Autodesk Fusion 360 part; units mm, degrees
sketch "Sketch1" plane through (0, 0, 0) normal (0, 0, 1) x (1, 0, 0)
  circle A0 centre (0, 0) radius 65
  dimension "d1" = 130
extrude "Extrude1" add sketch "Sketch1" along normal blind 60
hole "Hole1" at (0, 0, 60) direction (0, 0, -1) diameter 124 depth 55 tip angle 180
ref_plane "WorkPlane1" through (65, 0, 32.9588) normal (1, 0, 0) x (0, -1, 0)
ref_plane "WorkPlane2" through (77.5, 0, 32.9588) normal (1, 0, 0) x (0, -1, 0)
sketch "Sketch2" plane through (77.5, 0, 32.9588) normal (1, 0, 0) x (0, 1, 0)
  line L0 (-8, -8) -> (8, -8)
  line L1 (8, -8) -> (8, 18)
  line L2 (8, 18) -> (-8, 18)
  line L3 (-8, 18) -> (-8, -8)
  line L4 (-8, -8) -> (8, 18) construction
  line L5 (8, -8) -> (-8, 18) construction
  point P0 (0, 5)
  dimension "d9" = 16
extrude "Extrude2" add sketch "Sketch2" along normal up to surface end surface at (64.677, -6.4719, 40)
extrude "Extrude3" add 1 faces at (77.5, -2.6667, 33.6254) along direction (1, 0, 0) blind 0.5
extrude "Extrude4" cut 1 faces at (73.6667, 0, 24.9588) along direction (0, 0, 1) blind 1
extrude "Extrude5" add 1 faces at (78, -2.6667, 42.6254) along direction (1, 0, 0) blind 0.2
shell "Shell1" thickness 1 removed faces 2 at (69.0705, 8, 34.2921) at (73.8, 0, 50.9588)
ref_plane "WorkPlane3" through (49.7929, 41.7812, 24.979) normal (0.766, 0.6428, 0) x (0.6428, -0.766, 0)
sketch "Sketch3" plane through (49.7929, 41.7812, 24.979) normal (0.766, 0.6428, 0) x (0.6428, -0.766, 0)
  line L0 (20, -20) -> (-20, -20)
  line L1 (-20, -20) -> (-20, 10)
  line L2 (-20, 10) -> (20, 10)
  line L3 (20, 10) -> (20, -20)
  line L4 (20, -20) -> (-20, 10) construction
  line L5 (-20, -20) -> (20, 10) construction
  point P0 (0, -5)
  dimension "d20" = 40
extrude "Extrude6" cut sketch "Sketch3" against normal blind 20
fillet "Fillet1" radius 0.4 8 edges at (78.2, 0, 50.9588) (77.7, 8, 50.9588) (78.2, 8, 38.4588) (71.3529, 8, 25.9588) (78.2, 0, 25.9588) (78.2, -8, 38.4588) (71.3529, -8, 50.9588) (71.3529, -8, 25.9588)
fillet "Fillet2" radius 2 1 edges at (-60.6013, -23.505, 0)
ref_plane "WorkPlane4" through (49.7929, 41.7812, 24.979) normal (0.766, 0.6428, 0) x (0.6428, -0.766, 0)
ref_plane "WorkPlane5" through (-45.9619, -45.9619, 2.3267) normal (-0.7071, -0.7071, 0) x (-0.7071, 0.7071, 0)
ref_plane "WorkPlane6" through (-55.2958, -55.2958, 2.3267) normal (-0.7071, -0.7071, 0) x (-0.7071, 0.7071, 0)
sketch "Sketch4" plane through (-55.2958, -55.2958, 2.3267) normal (-0.7071, -0.7071, 0) x (-0.7071, 0.7071, 0)
  line L0 (13, -31.7116) -> (-13, -31.7116)
  line L1 (-13, -31.7116) -> (-13, -47.7116)
  line L2 (-13, -47.7116) -> (13, -47.7116)
  line L3 (13, -47.7116) -> (13, -31.7116)
  line L4 (13, -31.7116) -> (-13, -47.7116) construction
  line L5 (-13, -31.7116) -> (13, -47.7116) construction
  point P0 (0, -39.7116)
  dimension "d31" = 26
  dimension "d32" = 16
extrude "Extrude7" add sketch "Sketch4" along normal up to surface end surface at (62.1344, 19.0871, 28.7723)
extrude "Extrude8" cut 1 faces at (-52.2316, -58.3599, 39.3716) along direction (0.707107, 0.707107, 0) blind 0.5
shell "Shell2" thickness 1 removed faces 1 at (-52.9418, -50.8867, 50.0383)
Design review of the part built by this model. Coordinates are the model's own, in mm. A direction names the side the tool comes from. Round coordinates to 2 decimals unless told otherwise and drop trailing zeros. Write each loop counter-clockwise with the first axis right and the second up, starting at its lowest first coordinate (ties: lowest second). Pieces come first, ordered by that corner, then holes. Notation, with made-up numbers: (45.5, -7.75) -> (66.5, -7.75) arc R25 cw to (66.5, 11.25) -> close; hole circle Ø3 at (3, -13). An arc over 180 degrees is marked (long way). Answer in a Markdown table with one row per item.
Q1. Take a section at A-A, the plane y = 0. State the section outline as (x, z) points.
The answers:
| item | result |
|---|---|
| outline | (-65, 2) arc R2 ccw to (-63, 0) -> (63, 0) arc R2 ccw to (65, 2) -> (65, 25.96) -> (77.8, 25.96) arc R0.4 ccw to (78.2, 26.36) -> (78.2, 50.56) arc R0.4 ccw to (77.8, 50.96) -> (65, 50.96) -> (65, 60) -> (62, 60) -> (62, 5) -> (-62, 5) -> (-62, 60) -> (-65, 60) -> close |
Q2. Take a section at C-C, the plane x = 0. State the section outline as (y, z) points.
The answers:
| item | result |
|---|---|
| outline | (-65, 2) arc R2 ccw to (-63, 0) -> (63, 0) arc R2 ccw to (65, 2) -> (65, 60) -> (62, 60) -> (62, 5) -> (-62, 5) -> (-62, 60) -> (-65, 60) -> close |
Q3. Draft analysis for pull direction Y (two halves, no side actions). For faces 1 (the face through (71, 8, 38)), 2 (the face through (-1, 1, 5)), 3 (the face through (-59.25, -40.865, 42.15)), 4 (the face through (71, 0, 25.959)), state which applies: +Y half, -Y half, draft (parallel to the pull), parting line (faces both ways), or undercut.
The answers:
| item | result |
|---|---|
| face 1 | +Y half |
| face 2 | undercut |
| face 3 | undercut |
| face 4 | draft |
Q4. Clearance check with flat-ended pins moving along their axes: pin 1 Ø10 at (y, z) = (20, 19) entering from +X; pin 2 Ø4 at (x, z) = (72, 43) entering from -Y; pin 3 Ø3 at (y, z) = (-18.5, 42) entering from -X. State where each tip first meets the part, or that it passes through.
The answers:
| item | result |
|---|---|
| pin 1 | x = 63.25 |
| pin 2 | y = -8 |
| pin 3 | x = -62.74 |
Q5. For faces 5 (the face through (-40.865, -59.25, 41.926)), 6 (the face through (-50, -50, 50.038)), 7 (the face through (71, -8, 39)), list the 3-axis set-ups (+Z, -Z, +X, -X, +Y, -Y) from which the entire face can be reached by the end or side of a thin tool; tool diameter is ignored.
The answers:
| item | result |
|---|---|
| face 5 | +Z, -Z, -Y |
| face 6 | +Z, -X, -Y |
| face 7 | +Z, -Z, +X, -Y |
Q6. To check wall thickness, follow L1, parallel to Y at x = 0, z = 30; L2, parallel to Z at x = -15, y = 0. State the ranges of each line that lie inside material, in increasing order. Write a range as [from, to].
The answers:
| item | result |
|---|---|
| L1 | [-65, -62], [62, 65] |
| L2 | [0, 5] |
Q7. Take a section at D-D, the plane z = 56. State the section outline as (x, y) points.
The answers:
| item | result |
|---|---|
| outline | circle Ø130 at (0, 0); hole circle Ø124 at (0, 0) |
Q8. Take a section at B-B, the plane z = 40. State the section outline as (x, y) points.
The answers:
| item | result |
|---|---|
| outline | (-64.13, -45.75) -> (-45.75, -64.13) -> (-35.84, -54.23) arc R65 ccw to (64.51, -8) -> (77.8, -8) arc R0.4 ccw to (78.2, -7.6) -> (78.2, 7.6) arc R0.4 ccw to (77.8, 8) -> (64.51, 8) arc R65 ccw to (60.23, 24.43) -> (57.81, 22.4) arc R62 cw (long way) to (32.1, 53.04) -> (34.52, 55.08) arc R65 ccw to (-54.23, -35.84) -> close |
